Autodesk Inventor part; units mm, degrees
ref_plane "YZ Plane" through (0, 0, 0) normal (1, 0, 0) x (0, 1, 0)
ref_plane "XZ Plane" through (0, 0, 0) normal (0, 1, 0) x (-1, 0, 0)
ref_plane "XY Plane" through (0, 0, 0) normal (0, 0, 1) x (1, 0, 0)
sketch "スケッチ1" plane through (0, 0, 0) normal (0, 1, 0) x (-1, 0, 0)
  line L0 (3, 0) -> (6, 0)
  line L1 (6, 0) -> (6, 1.5)
  line L2 (6, 1.5) -> (5, 1.5)
  line L3 (5, 1.5) -> (5, 5)
  line L4 (4.5, 6) -> (3, 6)
  line L5 (3, 6) -> (3, 0)
  line L6 (5, 5) -> (4.5, 6)
  line L7 (0, -1.2) -> (0, 7.2)
  point P0 (0, 0)
  point P1 (3, 6)
  dimension "d5" = 1.5
  dimension "d9" = 1
  dimension "d10" = 0.5
  dimension "d17" = 10
  dimension "d18" = 12
  dimension "d19" = 6
  dimension "d20" = 6
revolve "回転1" add sketch "スケッチ1" angle 360 about axis through (0, 0, -10) along (0, 0, 1)
sketch "スケッチ2" plane through (0, 0, 6) normal (0, 0, 1) x (1, 0, 0)
  line L0 (4.4, -2.3749) -> (-4.4, -2.3749)
  line L1 (-4.4, -2.3749) -> (-4.4, 2.3749)
  line L2 (-4.4, 2.3749) -> (4.4, 2.3749)
  line L3 (4.4, 2.3749) -> (4.4, -2.3749)
  line L4 (4.4, -2.3749) -> (-4.4, 2.3749) construction
  line L5 (-4.4, -2.3749) -> (4.4, 2.3749) construction
  circle A0 centre (0, 0) radius 5
  point P0 (0, 0)
  dimension "d12" = 10
  dimension "d11" = 8.8
extrude "押し出し1" cut sketch "スケッチ2" against normal up to surface (4.5 mm away) contours L3 A0 | A0 L1
sketch "스케치3" plane through (0, 0, 6) normal (0, 0, 1) x (1, 0, 0)
  circle A0 centre (0, 0) radius 3
  line L0 (4.4, -0.9434) -> (4.4, 0.9434)
  arc A1 (4.4, 0.9434) -> (-4.4, 0.9434) centre (0, 0) ccw
  line L1 (-4.4, 0.9434) -> (-4.4, -0.9434)
  arc A2 (-4.4, -0.9434) -> (4.4, -0.9434) centre (0, 0) ccw
  circle A3 centre (0, 0) radius 3.025
  dimension "d21" = 6.05
extrude "돌출2" cut sketch "스케치3" against normal up to surface (6 mm away) contours A0 | A3
sketch "스케치4" plane through (0, 0, 6) normal (0, 0, 1) x (1, 0, 0)
  circle A0 centre (0, 0) radius 3.025
  line L0 (4.4, -0.9434) -> (4.4, 0.9434)
  arc A1 (4.4, 0.9434) -> (-4.4, 0.9434) centre (0, 0) ccw
  line L1 (-4.4, 0.9434) -> (-4.4, -0.9434)
  arc A2 (-4.4, -0.9434) -> (4.4, -0.9434) centre (0, 0) ccw
  line L2 (4.4, 0.9434) -> (4.4, 2.3749)
  arc A3 (4.4, 2.3749) -> (-4.4, 2.3749) centre (0, 0) ccw
  line L3 (-4.4, 2.3749) -> (-4.4, 0.9434)
  arc A4 (4.4, 0.9434) -> (-4.4, 0.9434) centre (0, 0) ccw
  line L4 (4.4, -2.3749) -> (4.4, -0.9434)
  arc A5 (-4.4, -0.9434) -> (4.4, -0.9434) centre (0, 0) ccw
  line L5 (-4.4, -0.9434) -> (-4.4, -2.3749)
  arc A6 (-4.4, -2.3749) -> (4.4, -2.3749) centre (0, 0) ccw
  arc A7 (4.375, 0.9407) -> (-4.375, 0.9407) centre (0, 0) ccw
  line L6 (4.375, 2.4206) -> (4.375, -2.4206)
  arc A8 (-4.375, -0.9407) -> (4.375, -0.9407) centre (0, 0) ccw
  line L7 (-4.375, -2.4206) -> (-4.375, 2.4206)
  point P0 (-4.35, 2.4653)
  point P1 (-4.35, -2.4653)
  point P2 (4.35, 2.4653)
  point P3 (4.35, -2.4653)
  point P4 (4.4, -0.9434)
  point P5 (4.4, 0.9434)
  point P6 (-4.4, 0.9434)
  point P7 (-4.4, -0.9434)
  point P8 (-4.4, 0.9434)
  point P9 (4.4, 0.9434)
  point P10 (-4.4, -0.9434)
  point P11 (4.4, -0.9434)
  dimension "d27" = 0.025
extrude "돌출3" cut sketch "스케치4" against normal up to surface (4.5 mm away) contours A2 L6 A1 L0 | L4 A6 L6 A2 | A1 L6 A3 L2 | L7 A6 L5 A2 | A2 L1 A1 L7 | A1 L3 A3 L7
properties part number "LED-0606" material "アセタール樹脂、黒"
Work out the finished part from the listing and answer in its coordinate system (mm). A direction names the side the tool comes from. Give positions to 0.01 mm unless a question says otherwise; leave off trailing zeros. Write each loop counter-clockwise with the first axis right and the second up, starting at its lowest first coordinate (ties: lowest second). Pieces come first, ordered by that corner, then holes.
(1) Flat-ended cylindrical pins translate along their axes: pin 1 Ø1.3 at (y, z) = (0.5, 2.5) entering from -X (3 decimals); pin 2 Ø1.5 at (y, z) = (3, 1) entering from -X; pin 3 Ø1.3 at (y, z) = (0.5, 3.5) entering from +X (3 decimals). Find the tip coordinate at first contact, or state that the pin passes through.
Final values:
pin 1: stops at x = -4.375
pin 2: stops at x = -5.56
pin 3: stops at x = 4.375
(2) Straight lines are drawn through the part: line 1 (Y direction, x = 0, z = 1.25) (3 decimals); line 2 (Y direction, x = 0, z = 4.2) (3 decimals); line 3 (Z direction, x = -1.25, y = 5). For each, find the intervals that lie inside material, in ascending order.
Final values:
line 1: y = -6 to -3.025, 3.025 to 6
line 2: y = -5 to -3.025, 3.025 to 5
line 3: z = 0 to 1.5
(3) The part is cut by section B-B on y = -0.5. Write down the section's boundary in (x, z) (3 decimals).
Final values:
outline: (-5.979, 0) - (-2.983, 0) - (-2.983, 6) - (-4.375, 6) - (-4.375, 1.5) - (-5.979, 1.5) - close; (2.983, 0) - (5.979, 0) - (5.979, 1.5) - (4.375, 1.5) - (4.375, 6) - (2.983, 6) - close
(4) The part is cut by section A-A on x = 0. Write down the section's boundary in (y, z) (3 decimals).
Final values:
outline: (-6, 0) - (-3.025, 0) - (-3.025, 6) - (-4.5, 6) - (-5, 5) - (-5, 1.5) - (-6, 1.5) - close; (3.025, 0) - (6, 0) - (6, 1.5) - (5, 1.5) - (5, 5) - (4.5, 6) - (3.025, 6) - close
(5) The part is cut by section C-C on z = 2. Write down the section's boundary in (x, y) (3 decimals), plus the area to 3 significant figures.
Final values:
outline: (-4.375, -2.421) arc R5 ccw to (4.375, -2.421) - (4.375, 2.421) arc R5 ccw to (-4.375, 2.421) - close; hole circle Ø6.05 at (0, 0)
area: 45.7 mm2
(6) The mould has two halves that part along Y. Classify faces 6 (the conical face through (0.1, -4.6, 5.8)), 7 (the conical face through (-0.1, 4.6, 5.8)), 8 (the cylindrical face through (2.794, -1.159, 3.042)): pulls with the +Y half, pulls with the -Y half, needs draft (parallel to the pull), parting line crosses it, or undercut.
Final values:
face 6: pulls with the -Y half
face 7: pulls with the +Y half
face 8: undercut
(7) The part is cut by section D-D on y = 5.5. Write down the section's boundary in (x, z).
Final values:
outline: (-2.4, 0) - (2.4, 0) - (2.4, 1.5) - (-2.4, 1.5) - close
(8) Which of the six approach directions +Z, -Z, +X, -X, +Y, -Y give full straight-line access (tool end or side, diameter ignored) to faces 1 (the cylindrical face through (0, 5, 3)), 2 (the cylindrical face through (6, 0, 1)), 3 (the cylindrical face through (0, -5, 3)), 4 (the flat face through (-4.375, 0, 4)), 5 (the flat face through (4.375, 0, 4))?
Final values:
face 1: +Z, +Y
face 2: +Z, -Z
face 3: +Z, -Y
face 4: +Z, -X, +Y, -Y
face 5: +Z, +X, +Y, -Y
